Part print with two shaded views. Sizes in mm from the minimum x, y, z corner. A direction names the side the tool comes from. Coordinates: 2 decimals unless noted, no trailing zeros. Write each loop counter-clockwise with the first axis right and the second up, starting at its lowest first coordinate (ties: lowest second). Pieces come first, ordered by that corner, then holes. Notation, with made-up numbers: (-14.5, 43) - (-5.5, 43) arc R8 ccw to (-5.5, 55) - close; hole circle Ø8 at (20.25, 8). An arc over 180 degrees is marked (long way). Answer in a Markdown table with one row per item. Add a question column.
Q1. Drill centre lines: line 1 along Y through (x, z) = (8, 4); line 2 along Y through (x, z) = (29.5, 9); line 3 along Z through (x, y) = (18.5, 8). Where is each one in solid material? Low to high. Write a range as from..to.
Q2. Band-saw the part on D-D (z = 8.25). List the corners of the cut face in (x, y), and give its area (3 significant figures).
Q3. Pin check, flat tips, straight feed: pin 1 (0.9 mm diameter, centred on x = 14.5, z = 11, fed in from +Y); pin 2 (1.5 mm diameter, centred on x = 4.5, y = 16, fed in from +Z); pin 3 (0.9 mm diameter, centred on y = 18.5, z = 11, fed in from +X). Stop position of each tip, or through.
Q4. Band-saw the part on B-B (x = 14). List the corners of the cut face in (y, z).
Q5. Band-saw the part on A-A (y = 5). List the corners of the cut face in (x, z), and give its area (3 significant figures).
Q6. Band-saw the part on C-C (z = 5.5). State how many separate pieces and enclosed holes the cut face has, and give its area (3 significant figures).
Q7. 3-axis set-ups, long thin cutter, end or side, ignore diameter. For the marked faces 1, 2 and 3: which of +Z, -Z, +X, -X, +Y, -Y reach the whole face in a straight line?
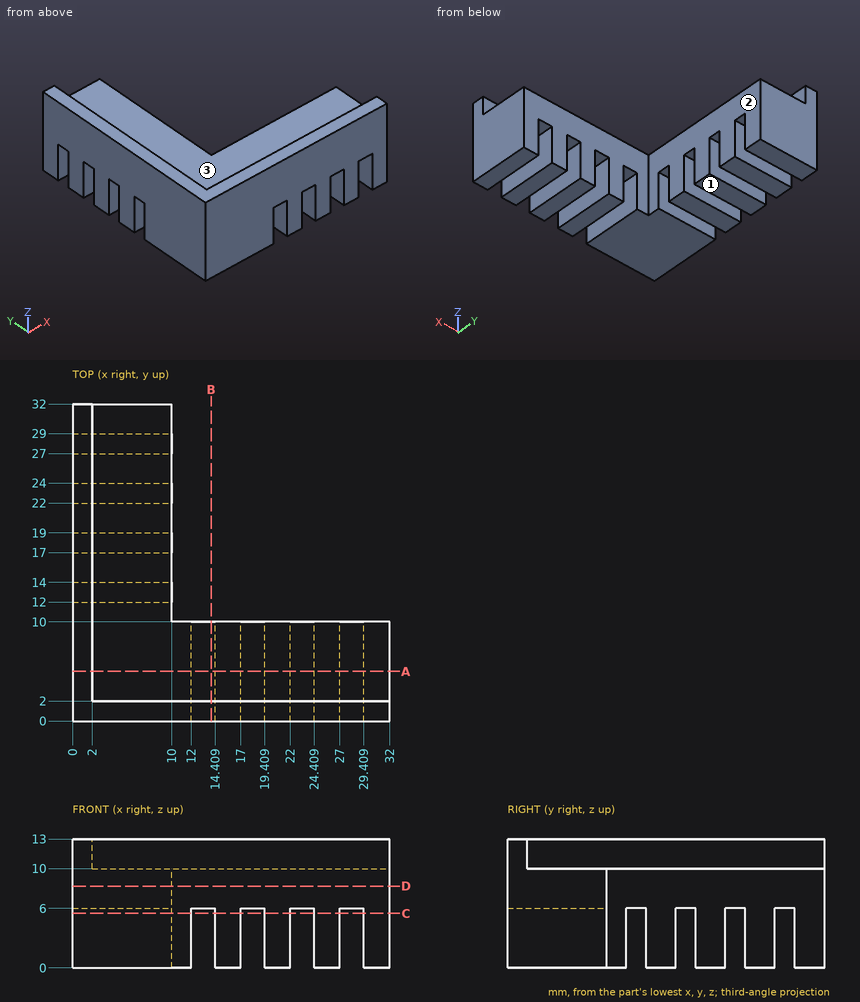
Checked values:
| question | item | result |
|---|---|---|
| 1 | line 1 | y = 0..12, 14..17, 19..22, 24..27, 29..32 |
| 1 | line 2 | y = 0..10 |
| 1 | line 3 | z = 6..10 |
| 2 | outline | (0, 0) - (32, 0) - (32, 10) - (10, 10) - (10, 32) - (0, 32) - close |
| 2 | area | 540 mm² |
| 3 | pin 1 | stops at y = 2 |
| 3 | pin 2 | stops at z = 10 |
| 3 | pin 3 | stops at x = 2 |
| 4 | outline | (0, 6) - (10, 6) - (10, 10) - (2, 10) - (2, 13) - (0, 13) - close |
| 5 | outline | (0, 0) - (12, 0) - (12, 6) - (14.41, 6) - (14.41, 0) - (17, 0) - (17, 6) - (19.41, 6) - (19.41, 0) - (22, 0) - (22, 6) - (24.41, 6) - (24.41, 0) - (27, 0) - (27, 6) - (29.41, 6) - (29.41, 0) - (32, 0) - (32, 10) - (2, 10) - (2, 13) - (0, 13) - close |
| 5 | area | 268 mm² |
| 6 | separate pieces | 9 |
| 6 | enclosed holes | 0 |
| 6 | area | 364 mm² |
| 7 | face 1 | -Z, +X, -X, +Y, -Y |
| 7 | face 2 | +Z, -Z, +X, +Y |
| 7 | face 3 | +Z, +X, +Y |
